Verification items for the finished model (mm, model axes). A direction names the side the tool comes from. Round coordinates to 2 decimals unless told otherwise and drop trailing zeros. Order: outer loops, then holes, each group sorted by start corner. A loop starts at its lowest first (then second) coordinate and runs counter-clockwise, first axis right, second up.
```python
from build123d import *

# Parameters (mm, degrees)
SKETCH_1_R          = 12.5
EXTRUDE_1_DEPTH     = 48.5
SKETCH_2_R          = 3.5
EXTRUDE_2_DEPTH     = 2.5
SKETCH_3_R          = 2
EXTRUDE_3_DEPTH     = 8
SKETCH_4_W          = 3.587297211
SKETCH_4_H          = 1.292719716
CUT_EXTRUDE_1_DEPTH = 8
SKETCH_5_R          = 1.5
CUT_EXTRUDE_2_DEPTH = 8
SKETCH_6_R          = 4
EXTRUDE_4_DEPTH     = 7.5
SKETCH_7_W          = 9
SKETCH_7_H          = 2
EXTRUDE_5_DEPTH     = 5


with BuildPart() as part:
    # 草图1 → 凸台-拉伸1 (new body)
    with BuildSketch(Plane.XY):
        with Locations(Location((0, 0, 0), (0, 0, 180))):
            Circle(SKETCH_1_R)
    extrude(amount=EXTRUDE_1_DEPTH)

    # 草图2 → 凸台-拉伸2 (add)
    with BuildSketch(Plane.XY.offset(48.5)):
        Circle(SKETCH_2_R)
    extrude(amount=EXTRUDE_2_DEPTH)

    # 草图3 → 凸台-拉伸3 (add)
    with BuildSketch(Plane.XY.offset(51)):
        Circle(SKETCH_3_R)
    extrude(amount=EXTRUDE_3_DEPTH)

    # 草图4 → 切除-拉伸1 (cut)
    with BuildSketch(Plane.XY.offset(59)):
        with Locations((0.022725356, 2.396212297)):
            Rectangle(SKETCH_4_W, SKETCH_4_H)
    extrude(amount=-CUT_EXTRUDE_1_DEPTH, mode=Mode.SUBTRACT)

    # 草图5 → 切除-拉伸2 (cut)
    with BuildSketch(Plane.XY.offset(48.5)):
        with Locations((4.996399446, -6.876481118)):
            Circle(SKETCH_5_R)
        with Locations((-6.876481118, -4.996399446)):
            Circle(SKETCH_5_R)
        with Locations((-4.996399446, 6.876481118)):
            Circle(SKETCH_5_R)
        with Locations((6.876481118, 4.996399446)):
            Circle(SKETCH_5_R)
    extrude(amount=-CUT_EXTRUDE_2_DEPTH, mode=Mode.SUBTRACT)

    # 草图6 → 凸台-拉伸4 (add)
    with BuildSketch(Plane(origin=(0, 0, 0), x_dir=(-1, 0, 0), z_dir=(0, 0, -1))):
        with Locations(Location((0, 0, 0), (0, 0, 180))):
            Circle(SKETCH_6_R)
    extrude(amount=EXTRUDE_4_DEPTH)

    # 草图7 → 凸台-拉伸5 (add)
    with BuildSketch(Plane(origin=(0, 0, 0), x_dir=(-1, 0, 0), z_dir=(0, 0, -1))):
        with Locations((0, 8)):
            Rectangle(SKETCH_7_W, SKETCH_7_H)
        with Locations((0, -8)):
            Rectangle(SKETCH_7_W, SKETCH_7_H)
    extrude(amount=EXTRUDE_5_DEPTH)


solid = part.part
```
1) Sectioned sample at D-D on z = 31.5. Record the cut outline in (x, y), then the cut area to 3 significant figures.
2) Sectioned sample at C-C on z = 53.5. Record the cut outline in (x, y).
3) Sectioned sample at B-B on x = 0. Record the cut outline in (y, z).
4) Go/stop test with flat-tipped pins: pin 1 Ø12 at (y, z) = (5, 49) entering from -X; pin 2 Ø1 at (x, z) = (-0.5, 54) entering from +Y; pin 3 Ø10 at (y, z) = (-6, 18.5) entering from +X; pin 4 Ø1 at (y, z) = (-6, 16.5) entering from +X (3 decimals). Record where each tip stops, or that it passes through.
5) Tool access check on faces 1 (the cylindrical face through (-4.3, 5.55, 44.56)), 2 (the flat face through (4.5, 8, -2)), 3 (the flat face through (0, 7, -2)). Record the directions out of +Z, -Z, +X, -X, +Y, -Y that give a thin tool (end or side, any length) a straight path to the whole face; none if there is none.
6) Scan lines: probe 1 along Z at (x, y) = (-0.5, -3.5); probe 2 along Z at (x, y) = (8.25, -7); probe 3 along Y at (x, z) = (-7, 46.5). Record each from-to range of solid material in increasing order.
7) Draft check along Y on faces 4 (the flat face through (0, 1.75, 55)), 5 (the cylindrical face through (-0.867, 3.905, -3.698)), 6 (the flat face through (0, 0, 59)). Enter one of: released by +Y, released by -Y, zero draft, split by the parting line, or undercut.
8) Sectioned sample at A-A on y = 0. Record the cut outline in (x, z).
Returned:
1. outline: circle Ø25 at (0, 0)
1. area: 491 mm2
2. outline: (-0.97, 1.75) arc R2 ccw (long way) to (0.97, 1.75) - close
3. outline: (-12.5, 0) - (-9, 0) - (-9, -5) - (-7, -5) - (-7, 0) - (-4, 0) - (-4, -7.5) - (4, -7.5) - (4, 0) - (7, 0) - (7, -5) - (9, -5) - (9, 0) - (12.5, 0) - (12.5, 48.5) - (3.5, 48.5) - (3.5, 51) - (1.75, 51) - (1.75, 59) - (-2, 59) - (-2, 51) - (-3.5, 51) - (-3.5, 48.5) - (-12.5, 48.5) - close
4. pin 1: stops at x = -12.5
4. pin 2: stops at y = 1.75
4. pin 3: stops at x = 12.46
4. pin 4: stops at x = 11.225
5. face 1: +Z
5. face 2: -Z, +X, +Y, -Y
5. face 3: -Z, +X, -X
6. probe 1: z = -7.5 to 48.5
6. probe 2: z = 0 to 48.5
6. probe 3: y = -10.36 to -6.49, -3.5 to 10.36
7. face 4: released by +Y
7. face 5: undercut
7. face 6: zero draft
8. outline: (-12.5, 0) - (-4, 0) - (-4, -7.5) - (4, -7.5) - (4, 0) - (12.5, 0) - (12.5, 48.5) - (3.5, 48.5) - (3.5, 51) - (2, 51) - (2, 59) - (-2, 59) - (-2, 51) - (-3.5, 51) - (-3.5, 48.5) - (-12.5, 48.5) - close
